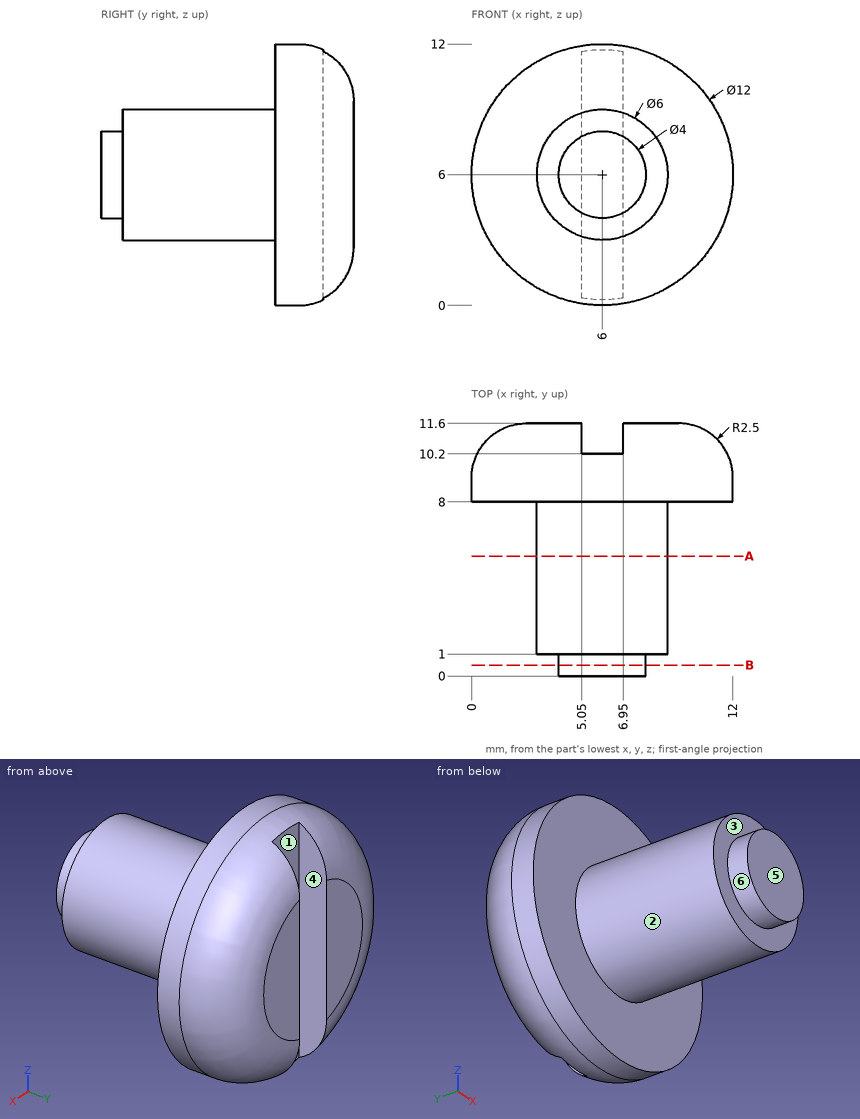
Design review of the part shown in the three views and the two pictorial views. Dimensions are in mm from the part's minimum x, y and z. A direction names the side the tool comes from. Round coordinates to 2 decimals unless told otherwise and drop trailing zeros. Loops run counter-clockwise (first coordinate to the right, second up) from the corner with the lowest first, then second, coordinate; pieces in that order, holes last.
1) Tool access review of the marked faces 5 and 6: name each direction out of +Z, -Z, +X, -X, +Y, -Y from which nothing blocks a thin tool from reaching the whole face with its end or side.
Values follow:
face 5: +Z, -Z, +X, -X, -Y
face 6: -Y
2) Consider section B-B on y = 0.5. State the section outline as (x, z) points, then the cut area to 3 significant figures.
Values follow:
outline: circle Ø4 at (6, 6)
area: 12.6 mm2
3) The part is to be moulded in two halves that separate along X. For the marked faces 1, 2, 3 and 4, say which applies: pulls with the +X half, pulls with the -X half, needs draft (parallel to the pull), parting line crosses it, or undercut.
Values follow:
face 1: undercut
face 2: parting line crosses it
face 3: needs draft
face 4: undercut
4) Wall thickness on line 1 along Y through (x, z) = (8, 7.5); line 2 along X through (y, z) = (10.25, 8.5); line 3 along Y through (x, z) = (5.25, 6.5): over which ranges is each line inside the solid? List them lowest first.
Values follow:
line 1: y = 1 to 11.6
line 2: x = 0.86 to 5.05, 6.95 to 11.14
line 3: y = 0 to 10.2
5) Clearance check with flat-ended pins moving along their axes: P1, Ø4, axis at x = 4.5, y = 2.5, coming from the +Z side; P2, Ø0.6, axis at x = 5.5, z = 3, coming from the +Y side; P3, Ø3, axis at x = 9, y = 7.5, coming from the -Z side. State where each tip first meets the part, or that it passes through.
Values follow:
P1: stops at z = 9
P2: stops at y = 10.2
P3: stops at z = 0.21
6) Consider section A-A on y = 5.5. State the section outline as (x, z) points, then the cut area to 3 significant figures.
Values follow:
outline: circle Ø6 at (6, 6)
area: 28.3 mm2
